Build history of the part. All positions in model axes, mm. A direction names the side the tool comes from. Coordinates: 2 decimals unless noted, no trailing zeros. Write each loop counter-clockwise with the first axis right and the second up, starting at its lowest first coordinate (ties: lowest second). Pieces come first, ordered by that corner, then holes.
```python
from build123d import *

# Parameters (mm, degrees)
SKETCH_1_R               = 15
SKETCH_1_R_2             = 7.2
EXTRUDE_1_DEPTH          = 8
CHAMFER_1_SIZE           = 0.5
CHAMFER_2_SIZE           = 2
EXTRUDE_2_DEPTH          = 1.5
PATTERN_CIRCULAR_1_COUNT = 3


with BuildPart() as part:
    # 草图1 → 凸台-拉伸1 (new body)
    with BuildSketch(Plane(origin=(0, 0, 0), x_dir=(1, 0, 0), z_dir=(0, 1, 0))):
        with Locations(Location((0, 0, 0), (0, 0, 270))):
            Circle(SKETCH_1_R)
        with Locations(Location((0, 0, 0), (0, 0, 270))):
            Circle(SKETCH_1_R_2, mode=Mode.SUBTRACT)
    extrude(amount=EXTRUDE_1_DEPTH)

    # 倒角1
    chamfer_1_edges = [part.edges().sort_by_distance(p)[0] for p in [
        (0, 0, -15),
    ]]
    chamfer(chamfer_1_edges, length=CHAMFER_1_SIZE)

    # 倒角2
    chamfer_2_edges = [part.edges().sort_by_distance(p)[0] for p in [
        (0, 0, -7.2),
    ]]
    chamfer(chamfer_2_edges, length=CHAMFER_2_SIZE)

    # 草图2 → 凸台-拉伸2 (add)
    with BuildSketch(Plane(origin=(0, 8, 0), x_dir=(1, 0, 0), z_dir=(0, 1, 0))):
        with BuildLine():
            Line((1.649657688, 9.355673654), (1.47600951, 8.370865901))
            ThreePointArc((1.47600951, 8.370865901), (0, 8.5), (-1.47600951, 8.370865901))
            Line((-1.47600951, 8.370865901), (-1.649657688, 9.355673654))
            ThreePointArc((-1.649657688, 9.355673654), (0, 9.5), (1.649657688, 9.355673654))
        make_face()
    extrude_2 = extrude(amount=EXTRUDE_2_DEPTH)

    # 阵列(圆周)1: 凸台-拉伸2 ×3 about axis
    pattern_circular_1_axis = Axis((0, 0, 0), (0, 1, 0))
    for i in range(1, PATTERN_CIRCULAR_1_COUNT):
        add(extrude_2.rotate(pattern_circular_1_axis, i * 360 / PATTERN_CIRCULAR_1_COUNT))


solid = part.part
```
1. Probe line 1 along X through (y, z) = (4.4, 0); line 2 along Y through (x, z) = (10.5, -9.5); line 3 along X through (y, z) = (2, 3.5). List the from-to ranges inside material, lowest first.
Computed values:
line 1: x = -15 to -7.2, 7.2 to 15
line 2: y = 0 to 8
line 3: x = -14.59 to -6.29, 6.29 to 14.59
2. Saw through at C-C on y = 5. List the corners of the cut face in (x, z), plus the area to 3 significant figures.
Computed values:
outline: circle Ø30 at (0, 0); hole circle Ø14.4 at (0, 0)
area: 544 mm2
3. 3-axis set-ups, long thin cutter, end or side, ignore diameter. For faces 1 (the face through (8.24, 8.74, 4.73)), 2 (the face through (-8.46, 8.74, 3.08)), 3 (the face through (8.451, 8.74, 3.076)), 4 (the face through (0, 8.7, -8.5)), 5 (the face through (-1.562, 8.74, -8.856)): which of +Z, -Z, +X, -X, +Y, -Y reach the whole face in a straight line?
Computed values:
face 1: +Z, +X, +Y
face 2: -Z, -X, +Y
face 3: -Z, +X, +Y
face 4: +Z, +Y
face 5: +Z, -X, +Y
4. Saw through at B-B on z = 0. List the corners of the cut face in (x, y).
Computed values:
outline: (-15, 0.5) - (-14.5, 0) - (-9.2, 0) - (-7.2, 2) - (-7.2, 8) - (-15, 8) - close; (7.2, 2) - (9.2, 0) - (14.5, 0) - (15, 0.5) - (15, 8) - (7.2, 8) - close
5. Saw through at A-A on x = 0. List the corners of the cut face in (y, z).
Computed values:
outline: (0, -14.5) - (0.5, -15) - (8, -15) - (8, -9.5) - (9.5, -9.5) - (9.5, -8.5) - (8, -8.5) - (8, -7.2) - (2, -7.2) - (0, -9.2) - close; (0, 9.2) - (2, 7.2) - (8, 7.2) - (8, 15) - (0.5, 15) - (0, 14.5) - close
6. Mould opens along X. For faces 6 (the face through (-2.76, 4.96, 6.65)), 7 (the face through (-8.2, 8.7, 4.8)), 8 (the face through (-8, 9.5, 4)) say: +X half, -X half, draft (parallel to the pull), parting line (faces both ways), or undercut.
Computed values:
face 6: undercut
face 7: -X half
face 8: draft
7. Saw through at D-D on y = 1.25. List the corners of the cut face in (x, z).
Computed values:
outline: circle Ø30 at (0, 0); hole circle Ø15.9 at (0, 0)
8. Flat gauge pins, fed straight in: pin 1 (5 mm diameter, centred on x = 5, y = 3.5, fed in from +Z); pin 2 (5 mm diameter, centred on y = 1.5, z = -6.5, fed in from +X); pin 3 (1 mm diameter, centred on x = 7.5, y = 5, fed in from -Z). Where does each tip first touch, or does it go through?
Computed values:
pin 1: stops at z = 14.79
pin 2: stops at x = 14.46
pin 3: stops at z = -13.27
